Source: CAD feature listing. Evaluate the final solid. Frame: model axes, mm. Face numbers are marked on the shaded views. A direction names the side the tool comes from. Give positions to 0.01 mm unless a question says otherwise; leave off trailing zeros. Order: outer loops, then holes, each group sorted by start corner. A loop starts at its lowest first (then second) coordinate and runs counter-clockwise, first axis right, second up. Notation, with made-up numbers: M 10,12.25 L 48,12.25 A26 cw 48,41.25 Z; hole C 85.25,32 d5. An arc over 180 degrees is marked long. One line per question, with ' | ' between items. Start each with the question number.
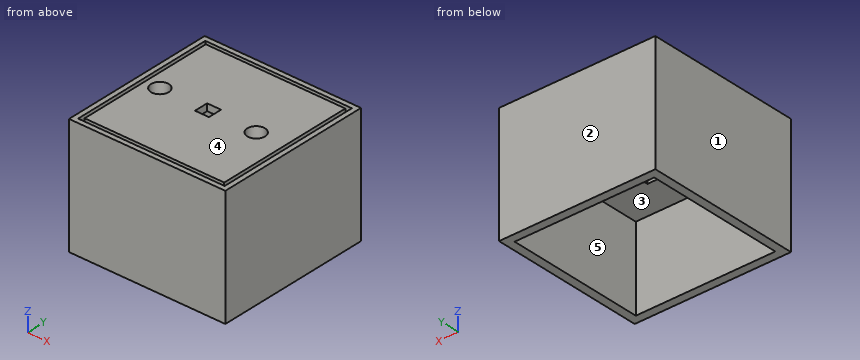
from build123d import *

# Parameters (mm, degrees)
SKETCH2_W           = 112
SKETCH2_H           = 112
SKETCH2_W_2         = 10
SKETCH2_H_2         = 10
BOSS_EXTRUDE1_DEPTH = 5
SKETCH3_W           = 112
SKETCH3_H           = 112
SKETCH3_W_2         = 105
SKETCH3_H_2         = 105
SKETCH3_W_3         = 100
SKETCH3_H_3         = 100
SKETCH3_R           = 6.35
SKETCH3_W_4         = 10
SKETCH3_H_4         = 10
BOSS_EXTRUDE2_DEPTH = 20
SKETCH4_W           = 50
SKETCH4_H           = 50
CUT_EXTRUDE1_DEPTH  = 20
SKETCH8_W           = 112
SKETCH8_H           = 112
SKETCH8_W_2         = 100
SKETCH8_H_2         = 100
BOSS_EXTRUDE3_DEPTH = 60


with BuildPart() as part:
    # Sketch2 → Boss-Extrude1 (new body)
    with BuildSketch(Plane.XY):
        Rectangle(SKETCH2_W, SKETCH2_H)
        with Locations((-5, 0)):
            Rectangle(SKETCH2_W_2, SKETCH2_H_2, mode=Mode.SUBTRACT)
    extrude(amount=BOSS_EXTRUDE1_DEPTH)

    # Sketch3 → Boss-Extrude2 (add)
    # profile 1 of 2: a face of its own
    with BuildSketch(Plane.XY.offset(5)):
        Rectangle(SKETCH3_W, SKETCH3_H)
        Rectangle(SKETCH3_W_2, SKETCH3_H_2, mode=Mode.SUBTRACT)
    # profile 2 of 2: a face of its own
    with BuildSketch(Plane.XY.offset(5)):
        Rectangle(SKETCH3_W_3, SKETCH3_H_3)
        with Locations((-39.5, 0)):
            Circle(SKETCH3_R, mode=Mode.SUBTRACT)
        with Locations((-5, 0)):
            Rectangle(SKETCH3_W_4, SKETCH3_H_4, mode=Mode.SUBTRACT)
        with Locations((29.5, 0)):
            Circle(SKETCH3_R, mode=Mode.SUBTRACT)
    extrude(amount=BOSS_EXTRUDE2_DEPTH)

    # Sketch4 → Cut-Extrude1 (cut)
    with BuildSketch(Plane(origin=(0, 0, 0), x_dir=(-1, 0, 0), z_dir=(0, 0, -1))):
        with Locations((5, 0)):
            Rectangle(SKETCH4_W, SKETCH4_H)
    extrude(amount=-CUT_EXTRUDE1_DEPTH, mode=Mode.SUBTRACT)

    # Sketch8 → Boss-Extrude3 (add)
    with BuildSketch(Plane(origin=(0, 0, 0), x_dir=(-1, 0, 0), z_dir=(0, 0, -1))):
        Rectangle(SKETCH8_W, SKETCH8_H)
        Rectangle(SKETCH8_W_2, SKETCH8_H_2, mode=Mode.SUBTRACT)
    extrude(amount=BOSS_EXTRUDE3_DEPTH)


solid = part.part
Item 1: Reachability of the marked faces 4 and 5 from +Z, -Z, +X, -X, +Y, -Y: full face, straight path, thin tool, end or side. Return the list, or none.
Item 2: Cut plane C-C on x = -39.5. Return the cut outline in (y, z).
Item 3: Cut plane B-B on z = -41. Return the cut outline in (x, y).
Item 4: Cut plane D-D on y = -13. Return the cut outline in (x, z).
Item 5: Pin query (flat end, axial travel): pin 1 Ø4 at (x, y) = (28.5, 0) entering from +Z; pin 2 Ø12 at (x, y) = (21.5, 43) entering from -Z. Return the tip coordinate at first contact, or that it passes through.
Item 6: Line query: line 1 (Y direction, x = -39.5, z = 20.5); line 2 (Y direction, x = -33, z = 10.5); line 3 (Y direction, x = 8.5, z = -24.5). Output: solid intervals per line, ascending.
Item 7: Mould query, pull axis Y, two halves, no side actions, for the marked faces 1, 2 and 3. Classes: pulls with the +Y half, pulls with the -Y half, needs draft (parallel to the pull), parting line crosses it, or undercut.
Results are:
1) face 4: +Z, +X, -X, +Y, -Y | face 5: -Z
2) outline: M -56,-60 L -50,-60 L -50,0 L 50,0 L 50,-60 L 56,-60 L 56,25 L 52.5,25 L 52.5,5 L 50,5 L 50,25 L 6.35,25 L 6.35,5 L -6.35,5 L -6.35,25 L -50,25 L -50,5 L -52.5,5 L -52.5,25 L -56,25 Z
3) outline: M -56,-56 L 56,-56 L 56,56 L -56,56 Z; hole M -50,-50 L 50,-50 L 50,50 L -50,50 Z
4) outline: M -56,-60 L -50,-60 L -50,0 L -30,0 L -30,20 L 20,20 L 20,0 L 50,0 L 50,-60 L 56,-60 L 56,25 L 52.5,25 L 52.5,5 L 50,5 L 50,25 L -50,25 L -50,5 L -52.5,5 L -52.5,25 L -56,25 Z
5) pin 1: stops at z = 5 | pin 2: stops at z = 0
6) line 1: y = -56 to -52.5, -50 to -6.35, 6.35 to 50, 52.5 to 56 | line 2: y = -56 to -52.5, -50 to 50, 52.5 to 56 | line 3: y = -56 to -50, 50 to 56
7) face 1: needs draft | face 2: pulls with the +Y half | face 3: undercut
